Verification items for the finished model (mm, model axes). A direction names the side the tool comes from. Round coordinates to 2 decimals unless told otherwise and drop trailing zeros. Write each loop counter-clockwise with the first axis right and the second up, starting at its lowest first coordinate (ties: lowest second). Pieces come first, ordered by that corner, then holes. Notation, with made-up numbers: M -7.5,28.5 L 50.5,28.5 A20 cw 50.5,53.5 Z; hole C 27,86.5 d9. An arc over 180 degrees is marked long. One line per item, written item: value. Start each with the question number.
Autodesk Inventor part; units mm, degrees
ref_plane "XZ Plane" through (0, 0, 0) normal (0, 1, 0) x (-1, 0, 0)
sketch "Sketch1" plane through (0, 0, 0) normal (0, 1, 0) x (-1, 0, 0)
  circle A0 centre (0, 0) radius 55
  circle A1 centre (0, 0) radius 50
  dimension "d0" = 110
  dimension "d1" = 100
extrude "Extrusion1" add sketch "Sketch1" along normal blind 30
ref_plane "Work Plane1" through (55, 0, 0) normal (1, 0, 0) x (0, 1, 0)
sketch "Sketch2" plane through (55, 0, 0) normal (1, 0, 0) x (0, 1, 0)
  line L0 (20, 5) -> (10, 5)
  line L1 (10, 5) -> (10, -5)
  line L2 (10, -5) -> (20, -5)
  line L3 (20, -5) -> (20, 5)
  line L4 (30, -55) -> (30, 55)
  line L5 (-6, 0) -> (36, 0)
  point P0 (0, 0)
  dimension "d5" = 10
  dimension "d6" = 10
  dimension "d7" = 10
  dimension "d8" = 5
extrude "Extrusion2" add sketch "Sketch2" along normal blind 20
extrude "Extrusion3" add sketch "Sketch2" against normal blind 5
properties part number "rim"
1) Mould release check, pull along X, two halves, no side actions. Record for faces 4 (the cylindrical face through (-47.69, 14.79, -15.02)), 5 (the cylindrical face through (-50.806, 14.79, 21.065)), 6 (the flat face through (75, 15, 0)), 7 (the flat face through (65, 20, 0)): pulls with the +X half, pulls with the -X half, needs draft (parallel to the pull), parting line crosses it, or undercut.
2) Cross-section at A-A (z = 0). Record the boundary of the cut face in (x, y).
3) Thickness scan on line 1 (Z direction, x = 0, y = 15.5); line 2 (X direction, y = 3.75, z = -28.5); line 3 (Z direction, x = 11.5, y = 26.5). Record the ranges inside material, lowest first.
4) Gauge pin test, flat ends, axial feed: pin 1 Ø3 at (x, y) = (-38, 22) entering from +Z; pin 2 Ø3 at (x, y) = (64, 13.5) entering from -Z; pin 3 Ø8 at (x, y) = (6.5, 24.5) entering from +Z. Record the tip position at first contact, or that the pin passes through.
5) Cross-section at C-C (x = 44). Record the boundary of the cut face in (y, z), then the cut area to 3 significant figures.
6) Cross-section at B-B (x = 0). Record the boundary of the cut face in (y, z).
7) Access from +Z, -Z, +X, -X, +Y, -Y to the whole of each face (thin tool, end or side, straight path). Record for faces 1 (the flat face through (65, 15, 5)), 2 (the flat face through (65, 15, -5)), 3 (the flat face through (-12, 0, -49)).
8) Cross-section at D-D (x = 61). Record the boundary of the cut face in (y, z), then the cut area to 3 significant figures.
Results below:
1. face 4: undercut
1. face 5: parting line crosses it
1. face 6: pulls with the +X half
1. face 7: needs draft
2. outline: M -55,0 L -50,0 L -50,30 L -55,30 Z; M 50,0 L 55,0 L 55,10 L 75,10 L 75,20 L 55,20 L 55,30 L 50,30 Z
3. line 1: z = -55 to -50, 50 to 55
3. line 2: x = -47.04 to -41.08, 41.08 to 47.04
3. line 3: z = -53.78 to -48.66, 48.66 to 53.78
4. pin 1: stops at z = 41.14
4. pin 2: stops at z = -5
4. pin 3: stops at z = 54.94
5. outline: M 0,-33 L 30,-33 L 30,-23.75 L 0,-23.75 Z; M 0,23.75 L 30,23.75 L 30,33 L 0,33 Z
5. area: 555 mm²
6. outline: M 0,-55 L 30,-55 L 30,-50 L 0,-50 Z; M 0,50 L 30,50 L 30,55 L 0,55 Z
7. face 1: +Z, +X, +Y, -Y
7. face 2: -Z, +X, +Y, -Y
7. face 3: +Z, -Z, +X, -X, -Y
8. outline: M 10,-5 L 20,-5 L 20,5 L 10,5 Z
8. area: 100 mm²
